Here's how the part is built. I have some questions about the finished solid (model axes, mm). Give positions to 0.01 mm unless a question says otherwise; leave off trailing zeros. Order: outer loops, then holes, each group sorted by start corner. A loop starts at its lowest first (then second) coordinate and runs counter-clockwise, first axis right, second up. Notation, with made-up numbers: (87.25, -16.75) - (112.25, -16.75) arc R11 ccw to (112.25, -10.75) - close; hole circle Ø9 at (8.5, -8). An arc over 180 degrees is marked (long way). One line per question, with ' | ' between items.
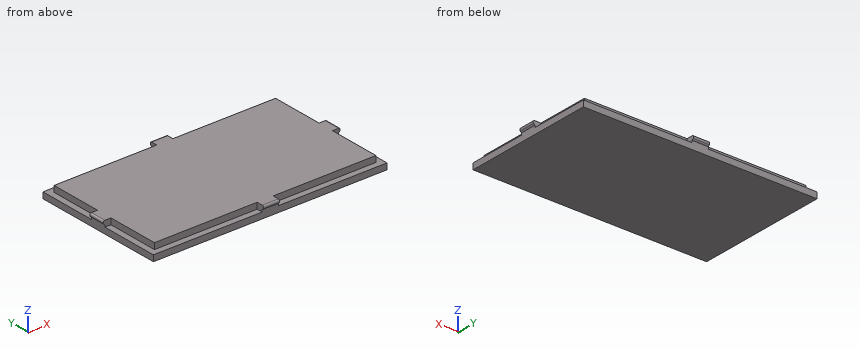
from build123d import *

# Parameters (mm, degrees)
F0_W      = 58
F0_H      = 33
F1_DEPTH  = 1.5
F2_W      = 55
F2_H      = 30
F3_DEPTH  = 1.5
F4_W      = 1.5
F4_H      = 4
F4_W_2    = 4
F4_H_2    = 1.5
F5_DEPTH  = 1.5
F7_DEPTH  = 4
F9_DEPTH  = 4
F11_DEPTH = 4
F13_DEPTH = 4
F14_R     = 0.4


with BuildPart() as f1:
    # F0 (on Top) → F1 (new body)
    with BuildSketch(Plane.XY):
        Rectangle(F0_W, F0_H)
    extrude(amount=F1_DEPTH)

    # F2 (on face) → F3 (join)
    with BuildSketch(Plane.XY.offset(1.5)):
        Rectangle(F2_W, F2_H)
    extrude(amount=F3_DEPTH)

    # F4 (on face) → F5 (join)
    with BuildSketch(Plane.XY.offset(1.5)):
        with Locations((-28.25, 0)):
            Rectangle(F4_W, F4_H)
        with Locations((0, 15.75)):
            Rectangle(F4_W_2, F4_H_2)
        with Locations((28.25, 0)):
            Rectangle(F4_W, F4_H)
        with Locations((0, -15.75)):
            Rectangle(F4_W_2, F4_H_2)
    extrude(amount=F5_DEPTH)

    # F6 (on face) → F7 (join)
    with BuildSketch(Plane(origin=(-2, 0, 0), x_dir=(0, -1, 0), z_dir=(-1, 0, 0))):
        Polygon((17.5, 3), (16.5, 3), (16.5, 2), align=None)
    extrude(amount=-F7_DEPTH)

    # F8 (on face) → F9 (join)
    with BuildSketch(Plane(origin=(0, 2, 0), x_dir=(-1, 0, 0), z_dir=(0, 1, 0))):
        Polygon((30, 3), (29, 3), (29, 2), align=None)
    extrude(amount=-F9_DEPTH)

    # F10 (on face) → F11 (join)
    with BuildSketch(Plane.XZ.offset(2)):
        Polygon((30, 3), (29, 3), (29, 2), align=None)
    extrude(amount=-F11_DEPTH)

    # F12 (on face) → F13 (join)
    with BuildSketch(Plane.YZ.offset(2)):
        Polygon((17.5, 3), (16.5, 3), (16.5, 2), align=None)
    extrude(amount=-F13_DEPTH)

    # F14
    f14_edges = [f1.edges().sort_by_distance(p)[0] for p in [
        (-30, 0, 3),
        (0, 17.5, 3),
        (30, 0, 3),
        (0, -17.5, 3),
    ]]
    fillet(f14_edges, radius=F14_R)


solid = f1.part
1) I want a section at A-A (y = -13). List the corners of the cut face in (x, z) for me.
Model answer:
outline: (-29, 0) - (29, 0) - (29, 1.5) - (27.5, 1.5) - (27.5, 3) - (-27.5, 3) - (-27.5, 1.5) - (-29, 1.5) - close
2) I want a section at B-B (x = -15.5). List the corners of the cut face in (y, z) for me.
Model answer:
outline: (-16.5, 0) - (16.5, 0) - (16.5, 1.5) - (15, 1.5) - (15, 3) - (-15, 3) - (-15, 1.5) - (-16.5, 1.5) - close
3) Please list where these lines run through material, in increasing order: L1, parallel to Y at x = 20.5, z = 1.4; L2, parallel to X at y = 8.5, z = 0.5; L3, parallel to Y at x = -26, z = 2.2.
Model answer:
L1: y = -16.5 to 16.5 | L2: x = -29 to 29 | L3: y = -15 to 15
4) I want a section at C-C (z = 0.75). List the corners of the cut face in (x, y) for me, plus the area to 3 significant figures.
Model answer:
outline: (-29, -16.5) - (29, -16.5) - (29, 16.5) - (-29, 16.5) - close | area: 1,910 mm2
5) I'm going to push flat-ended pins straight in: P1, Ø1.5, axis at y = -6, z = 1.5, coming from the +X side; P2, Ø1, axis at x = 7, z = 1, coming from the -Y side; P3, Ø1.6, axis at x = -28, z = 2.5, coming from the -Y side. Where does each tip first touch, or does it pass through?
Model answer:
P1: stops at x = 29 | P2: stops at y = -16.5 | P3: stops at y = -15
